Geometry: see drawing. Coordinates: mm, zero at the bounding-box minimum. A direction names the side the tool comes from. Give positions to 0.01 mm unless a question says otherwise; leave off trailing zeros. Write each loop counter-clockwise with the first axis right and the second up, starting at its lowest first coordinate (ties: lowest second). Pieces come first, ordered by that corner, then holes. Notation, with made-up numbers: (80, 61.25) - (120, 61.25) arc R29 cw to (120, 92.25) - close; hole circle Ø2 at (-9.5, 79). An arc over 180 degrees is marked (long way). Return JSON: item names as keys, results as strings.
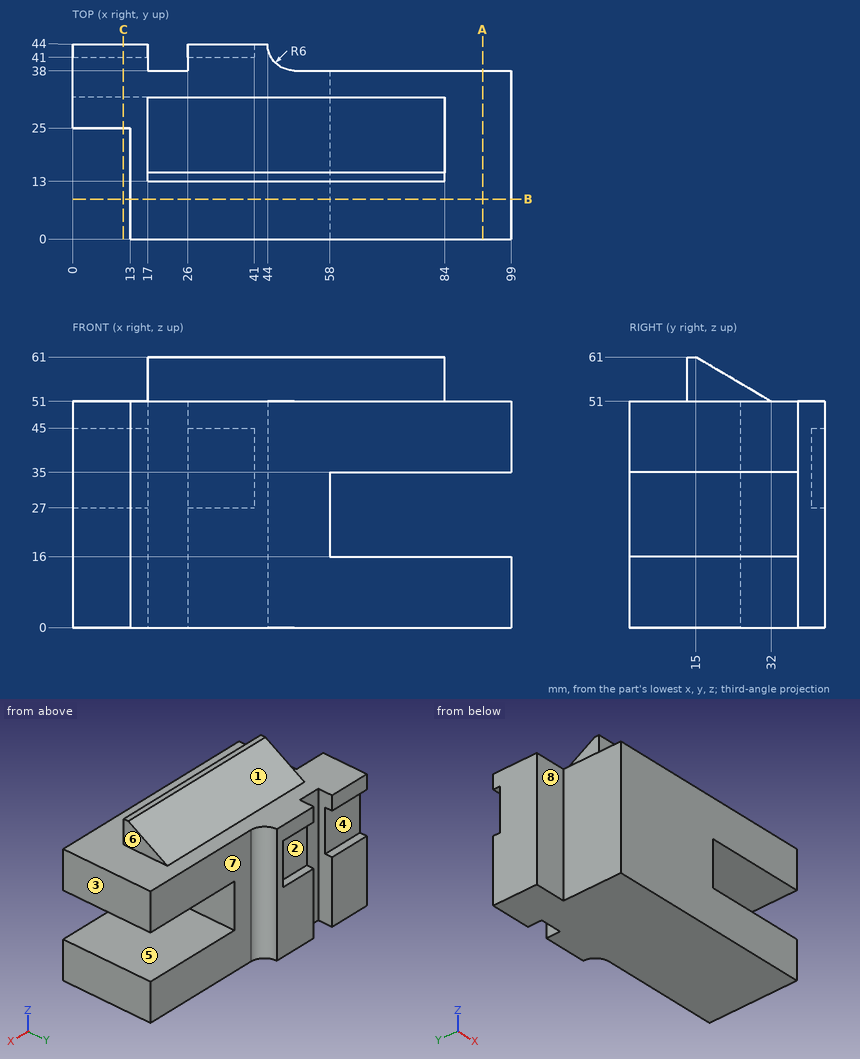
Q1. Pin query (flat end, axial travel): P1, Ø12, axis at x = 32, z = 36.5, coming from the +Y side; P2, Ø6.5, axis at x = 4, z = 13, coming from the -Y side; P3, Ø3, axis at x = 64.5, z = 57, coming from the -Y side; P4, Ø1, axis at x = 12, y = 7, coming from the +Z side. Return the tip coordinate at first contact, or that it passes through.
Answer key:
{"P1": "stops at y = 41", "P2": "stops at y = 25", "P3": "stops at y = 13", "P4": "passes through"}
Q2. Mould query, pull axis Z, two halves, no side actions, for the marked faces 1, 2 and 3. Classes: pulls with the +Z half, pulls with the -Z half, needs draft (parallel to the pull), parting line crosses it, or undercut.
Answer key:
{"face 1": "pulls with the +Z half", "face 2": "undercut", "face 3": "needs draft"}
Q3. Set-up query: the marked faces 4, 5, 6, 7 and 8. Return all of +Z, -Z, +X, -X, +Y, -Y with unobstructed straight access to the full face (end or side cutting, diameter ignored); none if empty.
Answer key:
{"face 4": "-X, +Y", "face 5": "+X, +Y, -Y", "face 6": "+Z, +X, +Y, -Y", "face 7": "+Z, -Z, +X, +Y", "face 8": "+Z, -Z, -X, -Y"}
Q4. Section query C-C, the plane x = 11.5. Return the cut outline in (y, z), plus the area to 3 significant figures.
Answer key:
{"outline": "(25, 0) - (44, 0) - (44, 27) - (41, 27) - (41, 45) - (44, 45) - (44, 51) - (25, 51) - close", "area": "915 mm^2"}
Q5. Section query B-B, the plane y = 9. Return the cut outline in (x, z).
Answer key:
{"outline": "(13, 0) - (99, 0) - (99, 16) - (58, 16) - (58, 35) - (99, 35) - (99, 51) - (13, 51) - close"}
Q6. Material intervals for probe 1 along Z at (x, y) = (83, 34); probe 2 along Z at (x, y) = (28.5, 42.5); probe 3 along Y at (x, z) = (24.5, 18), sorted ascending. Write a range as [from, to].
Answer key:
{"probe 1": "z = [0, 16], [35, 51]", "probe 2": "z = [0, 27], [45, 51]", "probe 3": "y = [0, 38]"}
Q7. Section query A-A, the plane x = 92.5. Return the cut outline in (y, z).
Answer key:
{"outline": "(0, 0) - (38, 0) - (38, 16) - (0, 16) - close; (0, 35) - (38, 35) - (38, 51) - (0, 51) - close"}
